Part model, mm, in its own coordinate system. A direction names the side the tool comes from. Round coordinates to 2 decimals unless told otherwise and drop trailing zeros. Write each loop counter-clockwise with the first axis right and the second up, starting at its lowest first coordinate (ties: lowest second). Pieces come first, ordered by that corner, then holes. Notation, with made-up numbers: M 18,-37 L 22,-37 A19 cw 22,-5 Z; hole C -16.5,77.5 d4. An arc over 180 degrees is marked long. Answer as a JSON object with one key per item and string values. Group by question number.
1. Two-plate mould, pull along Y, no slides. Class faces 4 (the face through (25, -23, 4)), 5 (the face through (-21.06, 17.43, 37.23)), 6 (the face through (-9.381, 22.008, 4.056)): +Y half, -Y half, draft (parallel to the pull), parting line (faces both ways), or undercut.
2. Band-saw the part on D-D, the plane x = 18. Write the cut outline in (y, z).
3. Drop flat-ended pins along their axis: pin 1 (10 mm diameter, centred on y = -5, z = 41.5, fed in from +X); pin 2 (4 mm diameter, centred on x = -12.5, y = 15, fed in from +Z). Give the stop position or say it passes through.
4. Band-saw the part on C-C, the plane z = 35. Write the cut outline in (x, y), plus the area to 3 significant figures.
5. Which spindle directions (+Z, -Z, +X, -X, +Y, -Y) get a long thin tool onto all of the face, cutting with end or side? Do faces 1 (the face through (-10.3, 0.4, 8)), 2 (the face through (15, -15, 4)), 3 (the face through (-9.381, -17.992, 4.056)). Say none if no direction does.
6. Band-saw the part on B-B, the plane x = 8.5. Write the cut outline in (y, z), plus the area to 3 significant figures.
7. Drill centre lines: line 1 (Y direction, x = -12, z = 5.75); line 2 (Y direction, x = 18, z = 5.5); line 3 (X direction, y = 20, z = 6). Where is each one in solid material? Low to high. Write a range as from..to.
8. Band-saw the part on A-A, the plane y = 20. Write the cut outline in (x, z).
from build123d import *

# Parameters (mm, degrees)
F1_DEPTH = 8
F0_W     = 8
F0_H     = 60
F2_DEPTH = 50
F4_D     = 6.6
F4_DEPTH = 17.25
F4_TIP   = 1.9828400428
F5_D     = 6.6
F5_DEPTH = 17.25
F5_TIP   = 1.9828400428


with BuildPart() as f1:
    # F0 (on Top) → F1 (new body)
    with BuildSketch(Plane.XY):
        with BuildLine():
            Line((-17, -30), (25, -30))
            Line((25, -30), (25, -15))
            Line((25, -15), (5, -15))
            ThreePointArc((5, -15), (-10, 0), (5, 15))
            Line((5, 15), (25, 15))
            Line((25, 15), (25, 30))
            Line((25, 30), (-17, 30))
            Line((-17, 30), (-17, -30))
        make_face()
    extrude(amount=F1_DEPTH)

    # F0 (on Top) → F2 (join)
    with BuildSketch(Plane.XY):
        with Locations((-21, 0)):
            Rectangle(F0_W, F0_H)
    extrude(amount=F2_DEPTH)

    # F4
    with Locations(Plane(origin=(0, 0, 0), x_dir=(1, 0, 0), z_dir=(0, 0, -1))):
        with Locations((18, 20), (-12, 20), (18, -20), (-12, -20)):
            Hole(F4_D / 2, depth=F4_DEPTH)
            with Locations((0, 0, -(F4_DEPTH + F4_TIP / 2))):  # 118° drill point
                Cone(0, F4_D / 2, F4_TIP, mode=Mode.SUBTRACT)

    # F5
    with Locations(Plane.YZ.offset(-17)):
        with Locations((-15, 35), (15, 35)):
            Hole(F5_D / 2, depth=F5_DEPTH)
            with Locations((0, 0, -(F5_DEPTH + F5_TIP / 2))):  # 118° drill point
                Cone(0, F5_D / 2, F5_TIP, mode=Mode.SUBTRACT)


solid = f1.part
Worked answers:
{
 "1": {"face 4": "draft", "face 5": "undercut", "face 6": "undercut"},
 "2": {"outline": "M -30,0 L -23.3,0 L -23.3,8 L -30,8 Z; M -16.7,0 L -15,0 L -15,8 L -16.7,8 Z; M 15,0 L 16.7,0 L 16.7,8 L 15,8 Z; M 23.3,0 L 30,0 L 30,8 L 23.3,8 Z"},
 "3": {"pin 1": "stops at x = -17", "pin 2": "stops at z = 8"},
 "4": {"outline": "M -25,-30 L -17,-30 L -17,-18.3 L -25,-18.3 Z; M -25,-11.7 L -17,-11.7 L -17,11.7 L -25,11.7 Z; M -25,18.3 L -17,18.3 L -17,30 L -25,30 Z", "area": "374 mm^2"},
 "5": {"face 1": "+Z, +X, +Y, -Y", "face 2": "+Z, -Z, +X", "face 3": "+Z, -Z"},
 "6": {"outline": "M -30,0 L -15,0 L -15,8 L -30,8 Z; M 15,0 L 30,0 L 30,8 L 15,8 Z", "area": "240 mm^2"},
 "7": {"line 1": "y = -30..-23.3, -16.7..16.7, 23.3..30", "line 2": "y = -30..-23.3, -16.7..-15, 15..16.7, 23.3..30", "line 3": "x = -25..-15.3, -8.7..14.7, 21.3..25"},
 "8": {"outline": "M -25,0 L -15.3,0 L -15.3,8 L -17,8 L -17,50 L -25,50 Z; M -8.7,0 L 14.7,0 L 14.7,8 L -8.7,8 Z; M 21.3,0 L 25,0 L 25,8 L 21.3,8 Z"}
}
